Autodesk Inventor part; units mm, degrees
ref_plane "Work Plane1" through (29, 0, 0) normal (0, -1, 0) x (1, 0, 0)
ref_plane "YZ Plane" through (0, 0, 0) normal (1, 0, 0) x (0, 1, 0)
ref_plane "XZ Plane" through (0, 0, 0) normal (0, 1, 0) x (-1, 0, 0)
sketch "Sketch1" plane through (0, 0, 0) normal (0, 0, 1) x (1, 0, 0)
  line L0 (-1.3333, 0) -> (30, 0)
  line L1 (30, 0) -> (30, 3)
  line L2 (30, 3) -> (12, 3)
  line L3 (12, 3) -> (11.3865, 3)
  line L4 (11.3865, 3) -> (0, 3)
  line L5 (0, 3) -> (0, 5)
  line L6 (0, 5) -> (-6, 5)
  line L7 (-6, 5) -> (-6, 2.8868)
  line L8 (-6, 2.8868) -> (-3, 2.8868)
  line L9 (-3, 2.8868) -> (-1.3333, 0)
  line L10 (-13.2, 0) -> (37.2, 0)
  line L11 (0, -1) -> (0, 6)
  line L12 (12, 3) -> (0, 3) construction
  dimension "d1" = 18
  dimension "d2" = 0.6136
  dimension "d3" = 6
  dimension "d4" = 3
  dimension "d5" = 60
  dimension "d6" = 6
  dimension "d7" = 6
  dimension "d8" = 5.7735
  dimension "d9" = 10
  dimension "d26" = 30
revolve "Body" add sketch "Sketch1" angle 360 about axis through (-1.3333, 0, 0) along (1, 0, 0)
sketch "Sketch2" plane through (-6, 0, 0) normal (-1, 0, 0) x (0, 0, 1)
  circle A0 centre (0, 0) radius 2.8868
  line L0 (0, -7) -> (0, 7)
  line L1 (-7, 0) -> (7, 0)
  line L2 (2.8868, 0) -> (1.4434, -2.5)
  line L3 (1.4434, -2.5) -> (-1.4434, -2.5)
  line L4 (-1.4434, -2.5) -> (-2.8868, 0)
  line L5 (-2.8868, 0) -> (-1.4434, 2.5)
  line L6 (-1.4434, 2.5) -> (1.4434, 2.5)
  line L7 (1.4434, 2.5) -> (2.8868, 0)
extrude "Slot" add sketch "Sketch2" against normal up to next contours L7 A0 | A0 L2 | L6 L0 A0 | A0 L0 L3 | L0 L6 A0 | A0 L3 L0 | L4 A0 | A0 L5
fillet "Fillet1" radius 0.6 1 edges at (-6, -5, 0)
thread "Thread"
chamfer "Chamfer1" distance 0.6135 distance2 0.6135 1 edges at (30, -3, 0) measured on face at (30, -0.301, -1.1526)
ref_plane "Work Plane1" through (29, 0, 0) normal (0, -1, 0) x (1, 0, 0)
fillet "Fillet2" radius 0.1 1 edges at (0, -3, 0)
equation "\"d1\" = GEL"
equation "\"d3\" = KOH"
equation "\"d4\" = INTI"
equation "\"d6\" = GD"
equation "\"d7\" = BDM"
equation "\"d8\" = 1.1547 * SW"
equation "\"d9\" = KOD"
equation "\"d26\" = NLG"
equation "\"d30\" = R"
equation "\"d17\" = RR"
equation "\"d13\" = GEL"
equation "\"d15\" = -0.5 * SPD + 0.5 * GD"
equation "\"d16\" = GUL"
equation "\"GD\" = NND"
equation "\"NLG\" = 30"
equation "\"GEL\" = 18"
equation "\"KOD\" = 10"
equation "\"KOH\" = NND"
equation "\"INTI\" = 3"
equation "\"GAL\" = 0.61345 * PTC"
equation "\"GUL\" = 0.61345 * PTC"
equation "\"BDM\" = NND"
equation "\"SW\" = 5"
equation "\"RR\" = 0.1 * NND"
equation "\"SPD\" = NND - 1.2269 * PTC"
equation "\"R\" = 0.1"
equation "\"PHH\" = 0.2"
equation "\"GD1\" = THREADDIA - 1.2269 * PTC"
equation "\"THREADDIA\" = 6"
equation "\"FAWI\" = 45deg"
equation "\"PTC\" = 1"
equation "\"KOH1\" = 5.4"
equation "\"NND\" = 6"
equation "\"TOA\" = 30deg"
equation "\"E0\" = 1.155 * SW"
properties part number "AS 1420 - 1973 - M6 x 30" material "Steel, Mild"
The listing builds one solid part. Answer for the finished solid, in the listing's coordinates (mm). A direction names the side the tool comes from. Coordinates: 2 decimals unless noted, no trailing zeros. Loops run counter-clockwise (first coordinate to the right, second up) from the corner with the lowest first, then second, coordinate; pieces in that order, holes last.
1) Flat-ended cylindrical pins translate along their axes: pin 1 Ø2 at (y, z) = (-3.5, 1.5) entering from +X; pin 2 Ø1.5 at (x, z) = (26.5, -2.5) entering from +Y; pin 3 Ø1 at (x, z) = (-2, -1) entering from +Y. Find the tip coordinate at first contact, or state that the pin passes through.
2) Find section A-A on x = 21.5. Write down the section's boundary in (y, z).
3) A tool of negligible diameter and unlimited length cuts with its end or side. For faces 4 (the face through (-4.411, -1.268, -2.155)), 5 (the face through (-6, -2, 2)), 6 (the face through (15, -3, 0)), from which of +Z, -Z, +X, -X, +Y, -Y can it reach the whole face along a straight path? Write none if from no direction.
4) Find the intervals of material crossed by L1, parallel to Z at x = 25, y = 0; L2, parallel to X at y = -0.5, z = -3.5; L3, parallel to Y at x = 7.5, z = -1.75, in increasing order.
5) Determine the mould class of faces 1 (the face through (-4, 2.5, 0)), 2 (the face through (-2.74, -1.08, 4.88)), 3 (the face through (0, 3.3, 0.1)) for opening direction Y: pulls with the +Y half, pulls with the -Y half, needs draft (parallel to the pull), parting line crosses it, or undercut.
Values:
1. pin 1: stops at x = 29.58
1. pin 2: stops at y = 2.44
1. pin 3: stops at y = 4.97
2. outline: circle Ø6 at (0, 0)
3. face 4: -X
3. face 5: +Z, -Z, -X, +Y, -Y
3. face 6: +X
4. L1: z = -3 to 3
4. L2: x = -6 to 0
4. L3: y = -2.44 to 2.44
5. face 1: undercut
5. face 2: parting line crosses it
5. face 3: needs draft
